from build123d import *

# Parameters (mm, degrees)
SKETCH1_R           = 7.5
BOSS_EXTRUDE1_DEPTH = 10
SKETCH2_R           = 6.25
CUT_EXTRUDE1_DEPTH  = 7.5
SKETCH3_R           = 6.225
BOSS_EXTRUDE2_DEPTH = 7
SKETCH4_R           = 5
CUT_EXTRUDE3_DEPTH  = 10.5


with BuildPart() as part:
    # Sketch1 → Boss-Extrude1 (new body)
    with BuildSketch(Plane(origin=(0, 0, 0), x_dir=(1, 0, 0), z_dir=(0, 1, 0))):
        with Locations(Location((0, 0, 0), (0, 0, 270))):
            Circle(SKETCH1_R)
    extrude(amount=BOSS_EXTRUDE1_DEPTH)

    # Sketch2 → Cut-Extrude1 (cut)
    with BuildSketch(Plane.XZ):
        with Locations(Location((0, 0, 0), (0, 0, 270))):
            Circle(SKETCH2_R)
    extrude(amount=-CUT_EXTRUDE1_DEPTH, mode=Mode.SUBTRACT)

    # Sketch3 → Boss-Extrude2 (add)
    with BuildSketch(Plane(origin=(0, 10, 0), x_dir=(1, 0, 0), z_dir=(0, 1, 0))):
        with Locations(Location((0, 0, 0), (0, 0, 270))):
            Circle(SKETCH3_R)
    extrude(amount=BOSS_EXTRUDE2_DEPTH)

    # Sketch4 → Cut-Extrude3 (cut)
    with BuildSketch(Plane(origin=(0, 17, 0), x_dir=(1, 0, 0), z_dir=(0, 1, 0))):
        with Locations(Location((0, 0, 0), (0, 0, 270))):
            Circle(SKETCH4_R)
    extrude(amount=-CUT_EXTRUDE3_DEPTH, mode=Mode.SUBTRACT)


solid = part.part
Part model, mm, in its own coordinate system. A direction names the side the tool comes from. Give positions to 0.01 mm unless a question says otherwise; leave off trailing zeros. Loops run counter-clockwise (first coordinate to the right, second up) from the corner with the lowest first, then second, coordinate; pieces in that order, holes last. Notation, with made-up numbers: M 74,-36 L 102,-36 A8 ccw 102,-25 Z; hole C -39.75,-13 d3. An arc over 180 degrees is marked long. Put each result on its own line as item: value. Start each with the question number.
1) Flat gauge pins, fed straight in: pin 1 (2 mm diameter, centred on x = 4, z = -2, fed in from -Y); pin 2 (1 mm diameter, centred on y = 5, z = 5.5, fed in from -X); pin 3 (4 mm diameter, centred on y = 11, z = -3.5, fed in from -X). Where does each tip first touch, or does it go through?
2) Saw through at D-D (x = -5.25). List the corners of the cut face in (y, z).
3) Saw through at A-A (z = 0). List the corners of the cut face in (x, y) (3 decimals).
4) Pull direction X, two halves, no side cores. Call faces 4 (the cylindrical face through (-3.79, 13.45, -4.94)), 5 (the flat face through (5.1, 17, 0.9)), 6 (the cylindrical face through (1.88, 3.7, -5.96)): +X half, -X half, draft (parallel to the pull), parting line (faces both ways), or undercut.
5) 3-axis set-ups, long thin cutter, end or side, ignore diameter. For faces 1 (the flat face through (6, 10, -3)), 2 (the flat face through (5, 7.5, -2)), 3 (the cylindrical face through (-4.88, 12.32, -1.08)): which of +Z, -Z, +X, -X, +Y, -Y reach the whole face in a straight line?
6) Probe probe 1 along X at (y, z) = (3.75, 0); probe 2 along Y at (x, z) = (-6, -1); probe 3 along Y at (x, z) = (-3.5, 5.5). List the from-to ranges inside material, lowest first.
7) Saw through at C-C (y = 12.75). List the corners of the cut face in (x, z) (3 decimals).
8) Saw through at B-B (x = 0). List the corners of the cut face in (y, z) (3 decimals), then the cut area to 3 significant figures.
Numbers:
1. pin 1: y = 7.5
1. pin 2: x = -5.59
1. pin 3: x = -7.29
2. outline: M 0,-5.36 L 10,-5.36 L 10,-3.34 L 17,-3.34 L 17,3.34 L 10,3.34 L 10,5.36 L 0,5.36 L 0,3.39 L 7.5,3.39 L 7.5,-3.39 L 0,-3.39 Z
3. outline: M -7.5,0 L -6.25,0 L -6.25,7.5 L -5,7.5 L -5,17 L -6.225,17 L -6.225,10 L -7.5,10 Z; M 5,7.5 L 6.25,7.5 L 6.25,0 L 7.5,0 L 7.5,10 L 6.225,10 L 6.225,17 L 5,17 Z
4. face 4: parting line
4. face 5: draft
4. face 6: undercut
5. face 1: +Y
5. face 2: -Y
5. face 3: +Y, -Y
6. probe 1: -7.5 to -6.25, 6.25 to 7.5
6. probe 2: 7.5 to 17
6. probe 3: 0 to 10
7. outline: C 0,0 d12.45; hole C 0,0 d10
8. outline: M 0,-7.5 L 10,-7.5 L 10,-6.225 L 17,-6.225 L 17,-5 L 7.5,-5 L 7.5,-6.25 L 0,-6.25 Z; M 0,6.25 L 7.5,6.25 L 7.5,5 L 17,5 L 17,6.225 L 10,6.225 L 10,7.5 L 0,7.5 Z
8. area: 48.4 mm^2
